Build history of the part. All positions in model axes, mm. Round coordinates to 2 decimals unless told otherwise and drop trailing zeros. Write each loop counter-clockwise with the first axis right and the second up, starting at its lowest first coordinate (ties: lowest second). Pieces come first, ordered by that corner, then holes. Notation, with made-up numbers: (23, -2) - (65, -2) arc R15 cw to (65, 2) - close; hole circle Ø9 at (31.25, 69.25). An arc over 180 degrees is marked (long way). Answer as a JSON object with one key per item and string values. Group by question number.
Item 1: Probe line 1 (X direction, y = -84, z = 20.5); line 2 (Z direction, x = -76.5, y = -32); line 3 (X direction, y = -82, z = -27). List the from-to ranges inside material, lowest first. Write a range as from..to.
Item 2: Slice it at B-B, the plane x = 123.5. List the corners of the cut face in (y, z), then the cut area to 3 significant figures.
Item 3: Slice it at C-C, the plane z = -3. List the corners of the cut face in (x, y), then the cut area to 3 significant figures.
Item 4: Flat gauge pins, fed straight in: pin 1 (8 mm diameter, centred on y = -45.5, z = 15.5, fed in from -X); pin 2 (3 mm diameter, centred on y = -78.5, z = 23.5, fed in from -X); pin 3 (3 mm diameter, centred on x = 44, z = -24.5, fed in from +Y); pin 4 (10 mm diameter, centred on y = -30.5, z = 26.5, fed in from -X). Where does each tip first touch, or does it go through?
from build123d import *

# Parameters (mm, degrees)
F1_DEPTH = 88.9


with BuildPart() as f1:
    # F0 (on Front) → F1 (new body)
    with BuildSketch(Plane.XZ):
        with BuildLine():
            Line((-152.4, -44.465989), (152.4, -44.465989))
            Line((152.4, -44.465989), (152.4, -44.434011))
            ThreePointArc((152.4, -44.434011), (137.521024, -8.512987), (101.6, 6.365989))
            ThreePointArc((101.6, 6.365989), (90.440768, 33.306757), (63.5, 44.465989))
            Line((63.5, 44.465989), (-63.5, 44.465989))
            ThreePointArc((-63.5, 44.465989), (-90.440768, 33.306757), (-101.6, 6.365989))
            ThreePointArc((-101.6, 6.365989), (-137.521024, -8.512987), (-152.4, -44.434011))
            Line((-152.4, -44.434011), (-152.4, -44.465989))
        make_face()
    extrude(amount=F1_DEPTH)


solid = f1.part
Geometry says:
{
 "1": {"line 1": "x = -98.88..98.88", "line 2": "z = -44.47..42.18", "line 3": "x = -149.31..149.31"},
 "2": {"outline": "(-88.9, -44.47) - (0, -44.47) - (0, 1.4) - (-88.9, 1.4) - close", "area": "4,080 mm^2"},
 "3": {"outline": "(-130.99, -88.9) - (130.99, -88.9) - (130.99, 0) - (-130.99, 0) - close", "area": "23,300 mm^2"},
 "4": {"pin 1": "stops at x = -101.25", "pin 2": "stops at x = -98.24", "pin 3": "stops at y = 0", "pin 4": "stops at x = -98.47"}
}
